from build123d import *

# Parameters (mm, degrees)
CUT_EXTRUDE1_START = 37.338
CUT_EXTRUDE1_DEPTH = 2.413


with BuildPart() as part:
    # Sketch2 → Revolve1 (revolve)
    with BuildSketch(Plane(origin=(0, 0, 0), x_dir=(0, 0, -1), z_dir=(1, 0, 0)), mode=Mode.PRIVATE) as revolve1_sk:
        with BuildLine():
            Line((37.338, 0), (37.338, 1.8176875))
            Line((37.338, 1.8176875), (36.7426875, 2.413))
            Line((36.7426875, 2.413), (-32.512, 2.413))
            Line((-32.512, 2.413), (-32.512, 3.72745))
            ThreePointArc((-32.512, 3.72745), (-32.582675134, 3.898074866), (-32.7533, 3.96875))
            Line((-32.7533, 3.96875), (-37.0967, 3.96875))
            ThreePointArc((-37.0967, 3.96875), (-37.267324866, 3.898074866), (-37.338, 3.72745))
            Line((-37.338, 3.72745), (-37.338, 0))
            Line((-37.338, 0), (37.338, 0))
        make_face()
    revolve(revolve1_sk.sketch.rotate(Axis((0, 0, -37.338), (0, 0, 1)), 90), axis=Axis((0, 0, -37.338), (0, 0, 1)))

    # Sketch3 → Cut-Extrude1 (cut)
    with BuildSketch(Plane.XY.offset(CUT_EXTRUDE1_START)):
        Polygon((-1.984375, 1.14567944), (-1.984375, -1.14567944), (0, -2.291358881), (1.984375, -1.14567944), (1.984375, 1.14567944), (0, 2.291358881), align=None)
    extrude(amount=-CUT_EXTRUDE1_DEPTH, mode=Mode.SUBTRACT)

    # Cut-Extrude2 cone 1 section (through the dimple's axis) → Cut-Extrude2 (revolve, cut)
    with BuildSketch(Plane(origin=(0, 0, 37.338), x_dir=(0, -1, 0), z_dir=(1, 0, 0))):
        Polygon((0, 0), (2.530707401, 0), (0, 1.461104599), align=None)
    revolve(axis=Axis((0, 0, 37.338), (0, 0, -1)), mode=Mode.SUBTRACT)


solid = part.part
Could you check a few things on this model? Use its own coordinates, in mm. A direction names the side the tool comes from. Round coordinates to 2 decimals unless told otherwise and drop trailing zeros. Order: outer loops, then holes, each group sorted by start corner. A loop starts at its lowest first (then second) coordinate and runs counter-clockwise, first axis right, second up.
Q1. Please list where these lines run through material, in increasing order: probe 1 along Y at (x, z) = (0.75, 24); probe 2 along Z at (x, y) = (-1, 2.5); probe 3 along Z at (x, y) = (-0.25, -1.25) (3 decimals).
Geometry says:
probe 1: y = -2.29 to 2.29
probe 2: z = 32.51 to 37.34
probe 3: z = -37.338 to 34.925
Q2. Imagine slicing it at B-B, the plane z = 5.5. List the corners of the cut face in (x, y) for me, then the cut area to 3 significant figures.
Geometry says:
outline: circle Ø4.83 at (0, 0)
area: 18.3 mm2
Q3. I'm going to push flat-ended pins straight in: P1, Ø2, axis at x = -0.5, y = -1, coming from the +Z side; P2, Ø2, axis at y = 0, z = 13.5, coming from the -X side; P3, Ø3, axis at x = -2, z = 29, coming from the -Y side. Where does each tip first touch, or does it pass through?
Geometry says:
P1: stops at z = 37.1
P2: stops at x = -2.41
P3: stops at y = -2.36
Q4. Which directions (+Z, -Z, +X, -X, +Y, -Y) give clear straight access to the entire face, cutting with the end or side of a thin tool? Please do faces 4 (the face through (0, -3, 37.338)), 5 (the face through (1.915, 1.468, -1.631)), 6 (the face through (-1.984, 0, 36)).
Geometry says:
face 4: +Z, +X, -X, +Y, -Y
face 5: -Z
face 6: +Z
Q5. Imagine slicing it at A-A, the plane y = 0. List the corners of the cut face in (x, z) for me (3 decimals).
Geometry says:
outline: (-3.969, 32.753) arc R0.241 ccw to (-3.727, 32.512) - (-2.413, 32.512) - (-2.413, -36.743) - (-1.818, -37.338) - (1.818, -37.338) - (2.413, -36.743) - (2.413, 32.512) - (3.727, 32.512) arc R0.241 ccw to (3.969, 32.753) - (3.969, 37.097) arc R0.241 ccw to (3.727, 37.338) - (2.531, 37.338) - (1.984, 37.023) - (1.984, 34.925) - (-1.984, 34.925) - (-1.984, 37.023) - (-2.531, 37.338) - (-3.727, 37.338) arc R0.241 ccw to (-3.969, 37.097) - close
Q6. Thinking about a two-plate mould opening in Y: for faces 1 (the face through (-0.978, 1.727, 36.078)), 2 (the face through (0.86, 3.874, 34.955)), 3 (the face through (0, 0, -37.338)), which applies, released by +Y, released by -Y, zero draft, split by the parting line, or undercut?
Geometry says:
face 1: undercut
face 2: split by the parting line
face 3: zero draft
